The model under review builds one solid part; all positions refer to its coordinate system, in mm. Round coordinates to 2 decimals unless told otherwise and drop trailing zeros. Order: outer loops, then holes, each group sorted by start corner. A loop starts at its lowest first (then second) coordinate and runs counter-clockwise, first axis right, second up. Notation, with made-up numbers: (56, 70.25) - (104, 70.25) arc R23 ccw to (104, 79.25) - close; hole circle Ø1 at (18.5, 81.5). An arc over 180 degrees is marked (long way). One line per question, with ' | ' between items. Start each with the question number.
Item 1: Insertion check: pin 1 Ø12 at (x, y) = (94, 4.5) entering from -Z; pin 2 Ø3 at (x, z) = (6.5, 3.5) entering from +Y. Each pin has a flat end and moves straight along its axis. Give the tip position at first contact, or say it passes through.
Item 2: Add section A-A on y = 8.75. State the section outline as (x, z) points (3 decimals).
Item 3: For L1, parallel to X at y = -2, z = 5.35; L2, parallel to X at y = 8.5, z = 0.3; L3, parallel to X at y = -9.25, z = 3.4, list the stretches that pass through material, from the lowest coordinate up. Write a range as [from, to].
Item 4: Add section B-B on z = 2.35. State the section outline as (x, y) points (3 decimals), and give its area (3 significant figures).
from build123d import *

# Parameters (mm, degrees)
SKETCH1_W           = 254
SKETCH1_H           = 50.8
BOSS_EXTRUDE1_DEPTH = 5.715
SKETCH2_W           = 10.16
SKETCH2_H           = 10.16
SKETCH2_W_2         = 12.7
SKETCH2_H_2         = 5.715
SKETCH2_W_3         = 38.1
CUT_EXTRUDE1_DEPTH  = 6.715
CUT_EXTRUDE2_DEPTH  = 6.715


with BuildPart() as part:
    # Sketch1 → Boss-Extrude1 (new body)
    with BuildSketch(Plane.XY):
        Rectangle(SKETCH1_W, SKETCH1_H)
    extrude(amount=BOSS_EXTRUDE1_DEPTH)

    # Sketch2 → Cut-Extrude1 (cut, through all)
    with BuildSketch(Plane.XY.offset(5.715)):
        with Locations((-58.42, 0)):
            Rectangle(SKETCH2_W, SKETCH2_H)
        with Locations((58.42, 0)):
            Rectangle(SKETCH2_W, SKETCH2_H)
        with Locations((0, -9.2075)):
            Rectangle(SKETCH2_W_2, SKETCH2_H_2)
        with Locations((0, 9.2075)):
            Rectangle(SKETCH2_W_3, SKETCH2_H_2)
    extrude(amount=-CUT_EXTRUDE1_DEPTH, mode=Mode.SUBTRACT)

    # Sketch3 → Cut-Extrude2 (cut, through all)
    with BuildSketch(Plane.XY.offset(5.715)):
        Polygon((-127, 25.4), (-127, 12.065), (-19.05, 12.065), (19.05, 12.065), (127, 12.065), (127, 25.4), align=None)
        Polygon((-6.35, -12.065), (-127, -12.065), (-127, -25.4), (127, -25.4), (127, -12.065), (6.35, -12.065), align=None)
    extrude(amount=-CUT_EXTRUDE2_DEPTH, mode=Mode.SUBTRACT)


solid = part.part
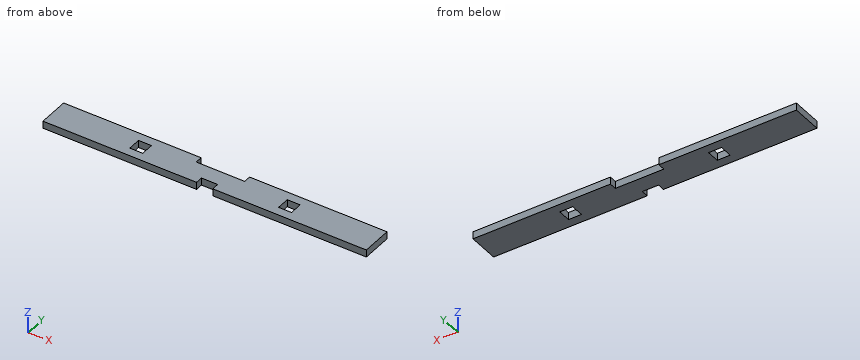
Determined:
1) pin 1: z = 0 | pin 2: y = 6.35
2) outline: (-127, 0) - (-19.05, 0) - (-19.05, 5.715) - (-127, 5.715) - close; (19.05, 0) - (127, 0) - (127, 5.715) - (19.05, 5.715) - close
3) L1: [-127, -63.5], [-53.34, 53.34], [63.5, 127] | L2: [-127, -19.05], [19.05, 127] | L3: [-127, -6.35], [6.35, 127]
4) outline: (-127, -12.065) - (-6.35, -12.065) - (-6.35, -6.35) - (6.35, -6.35) - (6.35, -12.065) - (127, -12.065) - (127, 12.065) - (19.05, 12.065) - (19.05, 6.35) - (-19.05, 6.35) - (-19.05, 12.065) - (-127, 12.065) - close; hole (-63.5, -5.08) - (-53.34, -5.08) - (-53.34, 5.08) - (-63.5, 5.08) - close; hole (53.34, -5.08) - (63.5, -5.08) - (63.5, 5.08) - (53.34, 5.08) - close | area: 5,630 mm2
